from build123d import *

# Parameters (mm, degrees)
ESBO_O2_W             = 1.5
ESBO_O2_H             = 7
CORTE_EXTRUS_O1_DEPTH = 0.5


with BuildPart() as part:
    # Esboço1 → Revolução1 (revolve)
    with BuildSketch(Plane(origin=(0, 0, 0), x_dir=(0, 0, -1), z_dir=(1, 0, 0)), mode=Mode.PRIVATE) as revolu_o1_sk:
        Polygon((0, 0), (0, 3.1475), (-1.56, 1.5875), (-11.56, 1.5875), (-11.56, 0), align=None)
    revolve(revolu_o1_sk.sketch.rotate(Axis((0, 0, 11.56), (0, 0, -1)), 180), axis=Axis((0, 0, 11.56), (0, 0, -1)))

    # Esboço2 → Corte-extrusão1 (cut)
    with BuildSketch(Plane(origin=(0, 0, 0), x_dir=(-1, 0, 0), z_dir=(0, 0, -1))):
        Rectangle(ESBO_O2_W, ESBO_O2_H)
    extrude(amount=-CORTE_EXTRUS_O1_DEPTH, mode=Mode.SUBTRACT)


solid = part.part
Check sheet for the modelled part. Datum: model origin and axes. Units: mm. A direction names the side the tool comes from. Coordinates: 2 decimals unless noted, no trailing zeros. Loops run counter-clockwise (first coordinate to the right, second up) from the corner with the lowest first, then second, coordinate; pieces in that order, holes last. Notation, with made-up numbers: (5.5, 31) -> (57.5, 31) arc R25 cw to (57.5, 48) -> close; hole circle Ø3 at (-18, 41.5). An arc over 180 degrees is marked (long way). Write item = value, one per line. Start each with the question number.
1. Section check A-A on y = 0. Record the cut outline in (x, z).
2. Section check B-B on x = 0. Record the cut outline in (y, z), then the cut area to 3 significant figures.
3. Section check D-D on z = 1. Record the cut outline in (x, y) (1 decimal).
4. Material ranges on line 1 (Z direction, x = 0.5, y = -0.25); line 2 (X direction, y = -0.5, z = 7.5); line 3 (Y direction, x = -0.25, z = 9.75), recorded low to high.
5. Section check C-C on z = 8. Record the cut outline in (x, y) (1 decimal), then the cut area to 3 significant figures.
6. Draft check along X on faces 1 (the flat face through (2, 0, 0)), 2 (the flat face through (0, 0, 0.5)), 3 (the conical face through (-0.552, -1.752, 1.311)). Enter one of: released by +X, released by -X, zero draft, split by the parting line, or undercut.
7. Depth check by flat-ended pin: P1, Ø1, axis at y = 0.5, z = 5.5, coming from the +X side; P2, Ø2, axis at x = -1, z = 6.5, coming from the -Y side. Enter the tip coordinate at first touch or a pass-through.
8. Tool access check on faces 4 (the cylindrical face through (1.41, -0.73, 6.63)), 5 (the flat face through (0, 0, 11.56)). Record the directions out of +Z, -Z, +X, -X, +Y, -Y that give a thin tool (end or side, any length) a straight path to the whole face; none if there is none.
Responses:
q1.outline = (-3.15, 0) -> (-0.75, 0) -> (-0.75, 0.5) -> (0.75, 0.5) -> (0.75, 0) -> (3.15, 0) -> (1.59, 1.56) -> (1.59, 11.56) -> (-1.59, 11.56) -> (-1.59, 1.56) -> close
q2.outline = (-2.65, 0.5) -> (2.65, 0.5) -> (1.59, 1.56) -> (1.59, 11.56) -> (-1.59, 11.56) -> (-1.59, 1.56) -> close
q2.area = 36.2 mm2
q3.outline = circle Ø4.3 at (0, 0)
q4.line_1 = 0.5 to 11.56
q4.line_2 = -1.51 to 1.51
q4.line_3 = -1.57 to 1.57
q5.outline = circle Ø3.2 at (0, 0)
q5.area = 7.92 mm2
q6.face_1 = zero draft
q6.face_2 = undercut
q6.face_3 = split by the parting line
q7.P1 = 1.59
q7.P2 = -1.59
q8.face_4 = +Z
q8.face_5 = +Z, +X, -X, +Y, -Y
